Geometry check sheet. Reference: the model listing, model coordinates, mm. Face numbers are marked on the shaded views. Coordinates: 2 decimals unless noted, no trailing zeros. Order: outer loops, then holes, each group sorted by start corner. A loop starts at its lowest first (then second) coordinate and runs counter-clockwise, first axis right, second up. Notation, with made-up numbers: (48.5, 23) - (77.5, 23) arc R8 cw to (77.5, 36) - close; hole circle Ø11 at (-18, 78.25). An arc over 180 degrees is marked (long way). One line per item, written item: value. Start each with the question number.
```python
from build123d import *

# Parameters (mm, degrees)
BOSS_EXTRUDE1_DEPTH  = 24
SKETCH2_R            = 2.05
CUT_EXTRUDE1_DEPTH   = 43.755116653
LPATTERN1_COUNT      = 3
LPATTERN1_PITCH      = 8
LPATTERN1_COUNT_DIR2 = 3
LPATTERN1_PITCH_DIR2 = 8
SKETCH3_R            = 2
CUT_EXTRUDE2_DEPTH   = 43.755116653
LPATTERN2_COUNT      = 3
LPATTERN2_PITCH      = 8
LPATTERN2_COUNT_DIR2 = 3
LPATTERN2_PITCH_DIR2 = 8
FILLET1_R            = 2


with BuildPart() as part:
    # Sketch1 → Boss-Extrude1 (new body)
    with BuildSketch(Plane.XY):
        Polygon((0, 0), (0, 26), (2, 26), (2, 2), (26, 2), (26, 0), align=None)
    extrude(amount=BOSS_EXTRUDE1_DEPTH)

    # Sketch2 → Cut-Extrude1 (cut, through all)
    with BuildSketch(Plane(origin=(2, 0, 0), x_dir=(0, 0, -1), z_dir=(1, 0, 0))):
        with Locations(Location((-20, 22, 0), (0, 0, 90))):
            Circle(SKETCH2_R)
    cut_extrude1 = extrude(amount=-CUT_EXTRUDE1_DEPTH, mode=Mode.SUBTRACT)

    # LPattern1: Cut-Extrude1 3 × 3
    with Locations(*[(0, -j * LPATTERN1_PITCH_DIR2, -i * LPATTERN1_PITCH) for i in range(LPATTERN1_COUNT) for j in range(LPATTERN1_COUNT_DIR2) if (i, j) != (0, 0)]):
        add(cut_extrude1, mode=Mode.SUBTRACT)

    # Sketch3 → Cut-Extrude2 (cut, through all)
    with BuildSketch(Plane(origin=(0, 2, 0), x_dir=(1, 0, 0), z_dir=(0, 1, 0))):
        with Locations(Location((22, -4, 0), (0, 0, 270))):
            Circle(SKETCH3_R)
    cut_extrude2 = extrude(amount=-CUT_EXTRUDE2_DEPTH, mode=Mode.SUBTRACT)

    # LPattern2: Cut-Extrude2 3 × 3
    with Locations(*[(-j * LPATTERN2_PITCH_DIR2, 0, i * LPATTERN2_PITCH) for i in range(LPATTERN2_COUNT) for j in range(LPATTERN2_COUNT_DIR2) if (i, j) != (0, 0)]):
        add(cut_extrude2, mode=Mode.SUBTRACT)

    # Fillet1
    fillet1_edges = [part.edges().sort_by_distance(p)[0] for p in [
        (1, 26, 24),
        (1, 26, 0),
        (26, 1, 24),
        (26, 1, 0),
    ]]
    fillet(fillet1_edges, radius=FILLET1_R)


solid = part.part
```
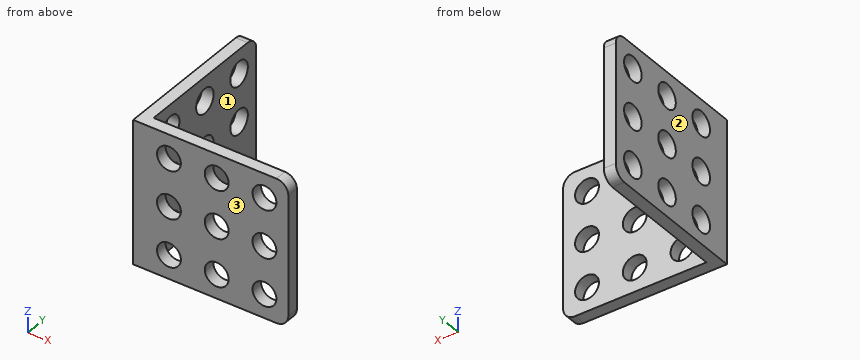
Q1. Material ranges on probe 1 along X at (y, z) = (0.5, 12); probe 2 along Z at (x, y) = (0.45, 22); probe 3 along X at (y, z) = (8, 11.25), recorded low to high.
Q2. Cross-section at C-C, the plane z = 21.5. Count the separate pieces of the cut face and the enclosed holes in it, and give its area (3 significant figures).
Q3. Cross-section at D-D, the plane z = 1.5. Enter the section's corners in (x, y).
Q4. Release check for a two-part mould opening along X. For the marked faces 1, 2 and 3 record: released by +X, released by -X, zero draft, split by the parting line, or undercut.
Q5. Cross-section at A-A, the plane y = 6. Enter the section's corners in (x, z).
Q6. Cross-section at B-B, the plane x = 22. Enter the section's corners in (y, z), and give its area (3 significant figures).
Q7. Gauge pin test, flat ends, axial feed: P1, Ø5.5, axis at y = 14, z = 4, coming from the +X side; P2, Ø12, axis at x = 19.5, z = 18.5, coming from the +Y side. Record the tip position at first contact, or that the pin passes through.
Check result:
1. probe 1: x = 0 to 4, 8 to 12, 16 to 20, 24 to 26
1. probe 2: z = 0 to 1.95, 6.05 to 9.95, 14.05 to 17.95, 22.05 to 24
1. probe 3: x = 0 to 2
2. separate pieces: 7
2. enclosed holes: 0
2. area: 67.4 mm2
3. outline: (0, 0) - (25.94, 0) - (25.94, 2) - (2, 2) - (2, 25.94) - (0, 25.94) - close
4. face 1: released by +X
4. face 2: released by -X
4. face 3: zero draft
5. outline: (0, 0) - (2, 0) - (2, 1.95) - (0, 1.95) - close; (0, 6.05) - (2, 6.05) - (2, 9.95) - (0, 9.95) - close; (0, 14.05) - (2, 14.05) - (2, 17.95) - (0, 17.95) - close; (0, 22.05) - (2, 22.05) - (2, 24) - (0, 24) - close
6. outline: (0, 0) - (2, 0) - (2, 2) - (0, 2) - close; (0, 6) - (2, 6) - (2, 10) - (0, 10) - close; (0, 14) - (2, 14) - (2, 18) - (0, 18) - close; (0, 22) - (2, 22) - (2, 24) - (0, 24) - close
6. area: 24.0 mm2
7. P1: stops at x = 2
7. P2: stops at y = 2
